Source: CAD feature listing. Evaluate the final solid. Frame: model axes, mm. Face numbers are marked on the shaded views. A direction names the side the tool comes from. Give positions to 0.01 mm unless a question says otherwise; leave off trailing zeros. Order: outer loops, then holes, each group sorted by start corner. A loop starts at its lowest first (then second) coordinate and runs counter-clockwise, first axis right, second up.
1) Access query for the marked faces 5 and 6. Directions: +Z, -Z, +X, -X, +Y, -Y. A direction counts if a zero-diameter tool reaches every point of the face in a straight line with its end or side. Return the directions, or none.
2) Section C-C, the plane x = -26.25. Return loops of the section in (y, z).
3) Draft query along X for the marked faces 1, 2, 3 and 4. Return one class per face: released by +X, released by -X, zero draft, split by the parting line, or undercut.
4) Section D-D, the plane z = 14.75. Return loops of the section in (x, y).
5) Material intervals for line 1 (X direction, y = 5, z = 2.5); line 2 (Y direction, x = -30.75, z = 6.25); line 3 (Y direction, x = -28, z = 10), sorted ascending.
6) Section A-A, the plane y = 4.75. Return loops of the section in (x, z).
7) First-contact query: P1, Ø2, axis at x = -29.5, z = 7.5, coming from the -Y side; P2, Ø2, axis at x = -24.5, z = 13.5, coming from the +Y side. Flat tips, straight axial feed; report the tip coordinate or a pass-through.
8) Section B-B, the plane x = -30.75. Return loops of the section in (y, z).
```python
from build123d import *

# Parameters (mm, degrees)
SKETCH2_R           = 5
BOSS_EXTRUDE1_DEPTH = 13
BOSS_EXTRUDE2_DEPTH = 4
SKETCH4_R           = 2.5
CUT_EXTRUDE1_DEPTH  = 13
SKETCH5_R           = 4
CUT_EXTRUDE2_DEPTH  = 4


with BuildPart() as part:
    # Sketch2 → Boss-Extrude1 (new body)
    with BuildSketch(Plane.XY):
        with Locations((-29.060949788, 5.337240829)):
            Circle(SKETCH2_R)
    extrude(amount=BOSS_EXTRUDE1_DEPTH)

    # Sketch3 → Boss-Extrude2 (add)
    with BuildSketch(Plane.XY.offset(13)):
        Polygon((-29.060949788, -1.590962401), (-23.060949788, 1.873139214), (-23.060949788, 8.801342444), (-29.060949788, 12.26544406), (-35.060949788, 8.801342444), (-35.060949788, 1.873139214), align=None)
    extrude(amount=BOSS_EXTRUDE2_DEPTH)

    # Sketch4 → Cut-Extrude1 (cut)
    with BuildSketch(Plane(origin=(0, 0, 0), x_dir=(-1, 0, 0), z_dir=(0, 0, -1))):
        with Locations((29.060949788, 5.337240829)):
            Circle(SKETCH4_R)
    extrude(amount=-CUT_EXTRUDE1_DEPTH, mode=Mode.SUBTRACT)

    # Sketch5 → Cut-Extrude2 (cut)
    with BuildSketch(Plane.XY.offset(17)):
        with Locations((-29.060949788, 5.337240829)):
            Circle(SKETCH5_R)
    extrude(amount=-CUT_EXTRUDE2_DEPTH, mode=Mode.SUBTRACT)


solid = part.part
```
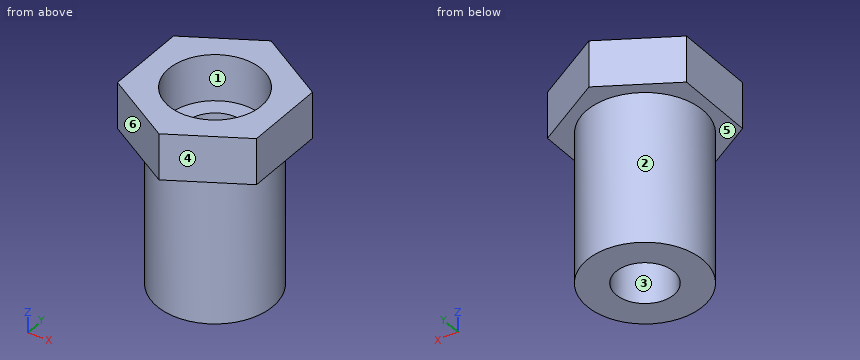
From the geometry:
1. face 5: -Z
1. face 6: +Z, -Z, -X, -Y
2. outline: (0.03, 13) - (1.2, 13) - (1.2, 0) - (9.47, 0) - (9.47, 13) - (10.64, 13) - (10.64, 17) - (8.18, 17) - (8.18, 13) - (2.49, 13) - (2.49, 17) - (0.03, 17) - close
3. face 1: undercut
3. face 2: split by the parting line
3. face 3: undercut
3. face 4: released by +X
4. outline: (-35.06, 1.87) - (-29.06, -1.59) - (-23.06, 1.87) - (-23.06, 8.8) - (-29.06, 12.27) - (-35.06, 8.8) - close; hole circle Ø8 at (-29.06, 5.34)
5. line 1: x = -34.05 to -31.54, -26.58 to -24.07
5. line 2: y = 0.63 to 3.49, 7.18 to 10.04
5. line 3: y = 0.45 to 3.07, 7.6 to 10.22
6. outline: (-35.06, 13) - (-34.03, 13) - (-34.03, 0) - (-31.49, 0) - (-31.49, 13) - (-33.02, 13) - (-33.02, 17) - (-35.06, 17) - close; (-26.63, 0) - (-24.1, 0) - (-24.1, 13) - (-23.06, 13) - (-23.06, 17) - (-25.1, 17) - (-25.1, 13) - (-26.63, 13) - close
7. P1: stops at y = 0.34
7. P2: stops at y = 10.21
8. outline: (-0.62, 13) - (0.63, 13) - (0.63, 0) - (3.49, 0) - (3.49, 13) - (1.71, 13) - (1.71, 17) - (-0.62, 17) - close; (7.18, 0) - (10.04, 0) - (10.04, 13) - (11.29, 13) - (11.29, 17) - (8.96, 17) - (8.96, 13) - (7.18, 13) - close
